Verification items for this drawing (mm, ordinates from the low corner). Coordinates: 2 decimals unless noted, no trailing zeros. Order: outer loops, then holes, each group sorted by start corner. A loop starts at its lowest first (then second) coordinate and runs counter-clockwise, first axis right, second up. Notation, with made-up numbers: M 25,-1 L 62,-1 A12 cw 62,8 Z; hole C 69,45 d4. An arc over 180 degrees is marked long. Write item = value, one per line.
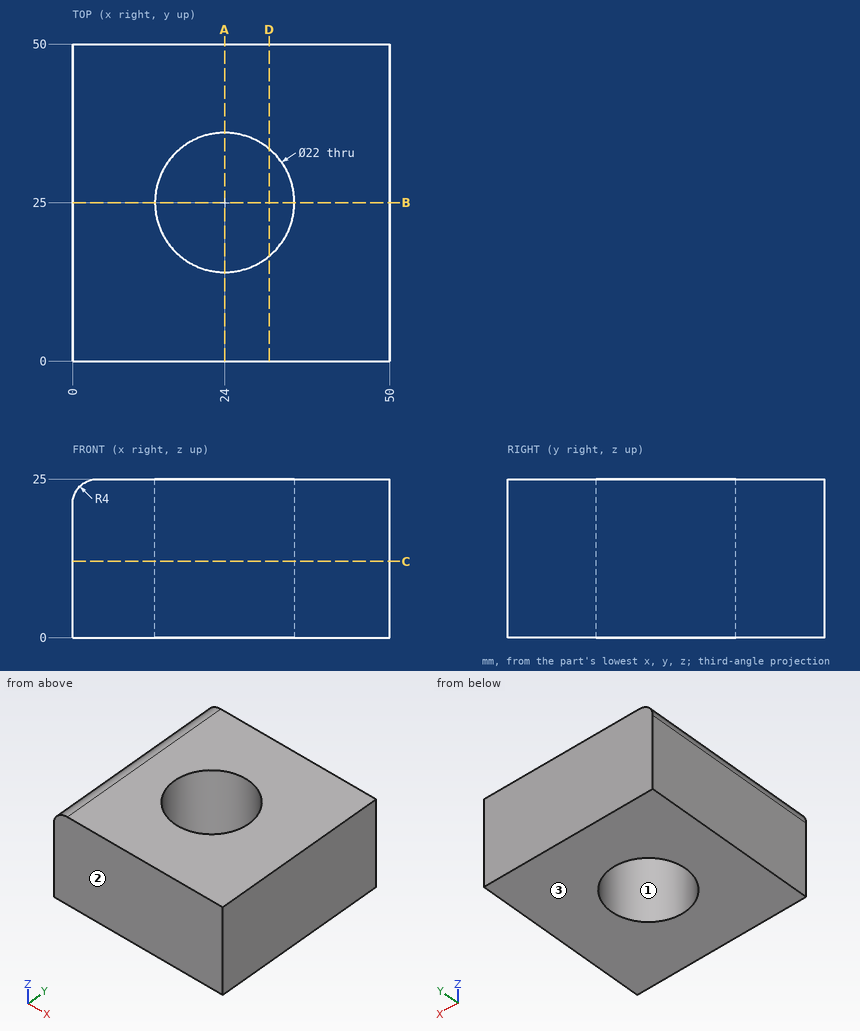
Item 1: Release check for a two-part mould opening along Y. For the marked faces 1, 2 and 3 record: pulls with the +Y half, pulls with the -Y half, needs draft (parallel to the pull), parting line crosses it, or undercut.
Report:
face_1 = undercut
face_2 = pulls with the -Y half
face_3 = needs draft
Item 2: Sectioned sample at D-D, the plane x = 31. Enter the section's corners in (y, z), then the cut area to 3 significant figures.
Report:
outline = M 0,0 L 16.51,0 L 16.51,25 L 0,25 Z; M 33.49,0 L 50,0 L 50,25 L 33.49,25 Z
area = 826 mm^2
Item 3: Sectioned sample at B-B, the plane y = 25. Enter the section's corners in (x, z), then the cut area to 3 significant figures.
Report:
outline = M 0,0 L 13,0 L 13,25 L 4,25 A4 ccw 0,21 Z; M 35,0 L 50,0 L 50,25 L 35,25 Z
area = 697 mm^2
Item 4: Sectioned sample at C-C, the plane z = 12. Enter the section's corners in (x, y), then the cut area to 3 significant figures.
Report:
outline = M 0,0 L 50,0 L 50,50 L 0,50 Z; hole C 24,25 d22
area = 2,120 mm^2
Item 5: Scan lines: L1, parallel to X at y = 24.5, z = 7.5; L2, parallel to Y at x = 24, z = 7.25; L3, parallel to Y at x = 26, z = 12. Record each from-to range of solid material in increasing order. Write a range as from..to.
Report:
L1 = 0..13.01, 34.99..50
L2 = 0..14, 36..50
L3 = 0..14.18, 35.82..50
Item 6: Sectioned sample at A-A, the plane x = 24. Enter the section's corners in (y, z), then the cut area to 3 significant figures.
Report:
outline = M 0,0 L 14,0 L 14,25 L 0,25 Z; M 36,0 L 50,0 L 50,25 L 36,25 Z
area = 700 mm^2
